```python
from build123d import *

# Parameters (mm, degrees)
BOSS_EXTRUDE1_DEPTH = 10
BOSS_EXTRUDE2_DEPTH = 1
CHAMFER1_SIZE       = 6
CHAMFER1_SIZE2      = 42.692218334
SKETCH3_R           = 1.75
CUT_EXTRUDE1_DEPTH  = 48.668671326
FILLET1_R           = 3


with BuildPart() as part:
    # Sketch1 → Boss-Extrude1 (new body, symmetric)
    with BuildSketch(Plane.XY):
        Polygon((-7.502714215, -23.495815343), (-9.382099457, -22.811775057), (7.71890771, 24.172855983), (22.71890771, 24.172855983), (22.71890771, 22.172855983), (9.119322786, 22.172855983), align=None)
    extrude(amount=BOSS_EXTRUDE1_DEPTH, both=True)

    # Sketch2 → Boss-Extrude2 (add)
    with BuildSketch(Plane.XY):
        Polygon((22.71890771, 22.172855983), (0.808304286, -0.66147968), (9.119322786, 22.172855983), align=None)
    extrude(amount=BOSS_EXTRUDE2_DEPTH)

    # Chamfer1
    chamfer1_edges = [part.edges().sort_by_distance(p)[0] for p in [
        (-8.442406836, -23.1537952, 10),
        (-8.442406836, -23.1537952, -10),
    ]]
    chamfer1_side = [part.faces().sort_by_distance(p)[0] for p in [
        (-8.442406836, -23.1537952, 0),
    ]]
    chamfer(chamfer1_edges, length=CHAMFER1_SIZE, length2=CHAMFER1_SIZE2, reference=chamfer1_side[0])

    # Sketch3 → Cut-Extrude1 (cut, through all)
    with BuildSketch(Plane(origin=(0, 24.172855983, 0), x_dir=(1, 0, 0), z_dir=(0, 1, 0))):
        with Locations((15, 6.365)):
            Circle(SKETCH3_R)
        with Locations((15, -6.365)):
            Circle(SKETCH3_R)
    extrude(amount=-CUT_EXTRUDE1_DEPTH, mode=Mode.SUBTRACT)

    # Fillet1
    fillet1_edges = [part.edges().sort_by_distance(p)[0] for p in [
        (22.71890771, 23.172855983, 10),
        (22.71890771, 23.172855983, -10),
    ]]
    fillet(fillet1_edges, radius=FILLET1_R)


solid = part.part
```
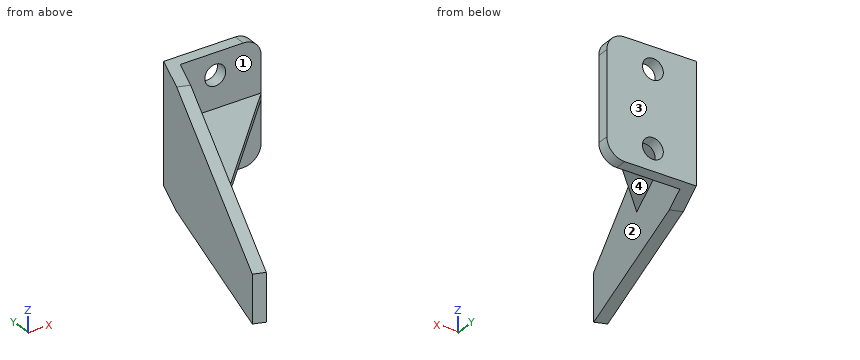
Check sheet for the modelled part. Datum: model origin and axes. Units: mm. Face numbers are marked on the shaded views. A direction names the side the tool comes from. Round coordinates to 2 decimals unless told otherwise and drop trailing zeros. Order: outer loops, then holes, each group sorted by start corner. A loop starts at its lowest first (then second) coordinate and runs counter-clockwise, first axis right, second up. Notation, with made-up numbers: (44, 82) -> (93, 82) arc R21 cw to (93, 112) -> close; hole circle Ø8 at (-28.75, -29). An arc over 180 degrees is marked (long way). One line per item, written item: value. Start each with the question number.
Q1. Gauge pin test, flat ends, axial feed: pin 1 Ø1 at (y, z) = (7, 5.5) entering from -X; pin 2 Ø5 at (x, y) = (12, 9) entering from -Z; pin 3 Ø8 at (y, z) = (18, -5.5) entering from +X. Record the tip position at first contact, or that the pin passes through.
Q2. Cross-section at B-B (x = 15). Record the boundary of the cut face in (y, z) (3 decimals), and give its area (3 significant figures).
Q3. Cross-section at A-A (z = 5.5). Record the boundary of the cut face in (x, y), and give its area (3 significant figures).
Q4. Cross-section at D-D (z = 2). Record the boundary of the cut face in (x, y).
Q5. Thickness scan on line 1 (Z direction, x = 15, y = 22.8) (3 decimals); line 2 (Y direction, x = 13.5, z = -4.25); line 3 (X direction, y = 22.5, z = -4.25). Record the ranges inside material, lowest first.
Q6. Cross-section at C-C (y = 20.5). Record the boundary of the cut face in (x, z).
Q7. Set-up check for the marked faces 1, 2, 3 and 4: record each of +Z, -Z, +X, -X, +Y, -Y from which the full face is reachable in a straight line by a thin tool's end or side.
Completed:
1. pin 1: stops at x = 1.29
1. pin 2: stops at z = 0
1. pin 3: stops at x = 9.06
2. outline: (14.129, 0) -> (22.173, 0) -> (22.173, -4.615) -> (24.173, -4.615) -> (24.173, 4.615) -> (22.173, 4.615) -> (22.173, 1) -> (14.129, 1) -> close; (22.173, -10) -> (24.173, -10) -> (24.173, -8.115) -> (22.173, -8.115) -> close; (22.173, 8.115) -> (24.173, 8.115) -> (24.173, 10) -> (22.173, 10) -> close
2. area: 34.0 mm²
3. outline: (-5.73, -12.78) -> (-3.85, -13.47) -> (9.12, 22.17) -> (13.48, 22.17) -> (13.48, 24.17) -> (7.72, 24.17) -> close; (16.52, 22.17) -> (22.72, 22.17) -> (22.72, 24.17) -> (16.52, 24.17) -> close
3. area: 99.8 mm²
4. outline: (-9.38, -22.81) -> (-7.5, -23.5) -> (9.12, 22.17) -> (22.72, 22.17) -> (22.72, 24.17) -> (7.72, 24.17) -> close
5. line 1: z = -10 to -8.115, -4.615 to 4.615, 8.115 to 10
5. line 2: y = 22.17 to 24.17
5. line 3: x = 7.11 to 22.72
6. outline: (6.38, -10) -> (8.51, -10) -> (8.51, 0) -> (21.11, 0) -> (21.11, 1) -> (8.51, 1) -> (8.51, 10) -> (6.38, 10) -> close
7. face 1: +Z, +X, -Y
7. face 2: +X, -Y
7. face 3: +Z, -Z, +X, -X, +Y
7. face 4: -Z, +X, -Y
